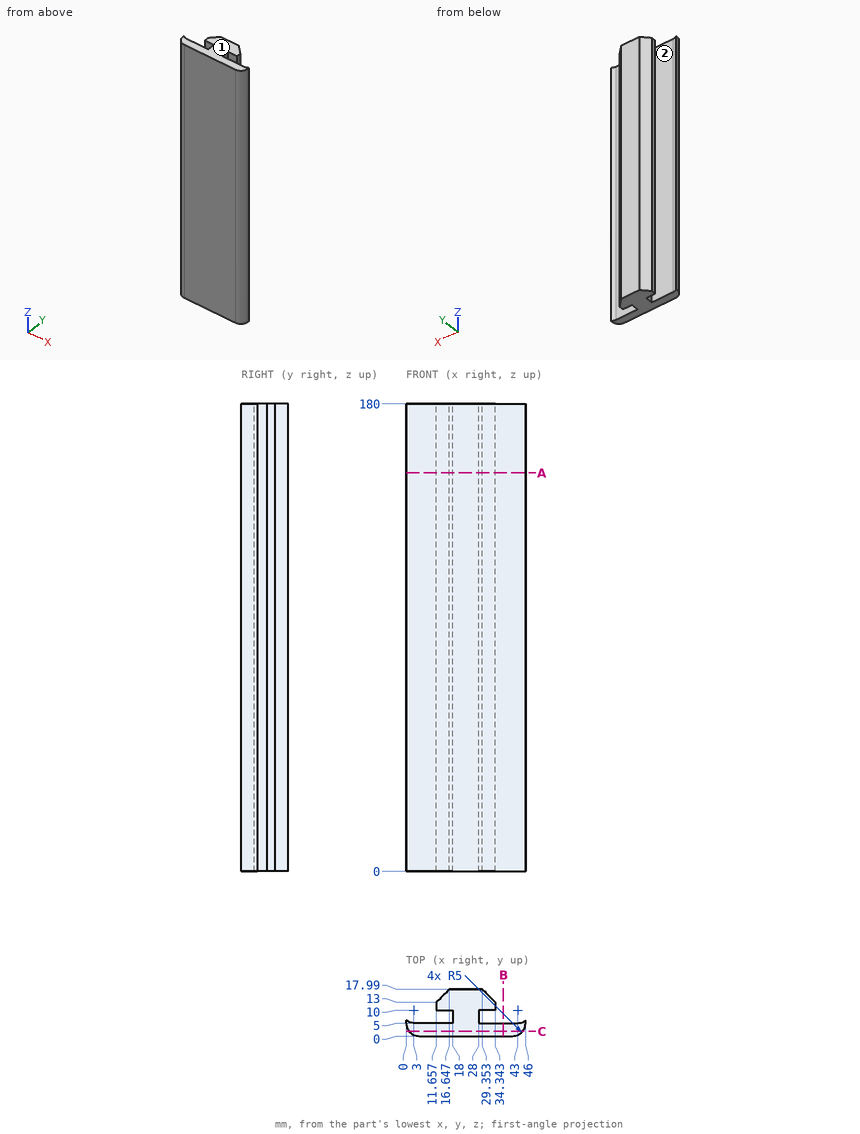
Source: three-view drawing plus pictorial views. Frame: mm from the lowest corner of the part. Round coordinates to 2 decimals unless told otherwise and drop trailing zeros. Loops run counter-clockwise (first coordinate to the right, second up) from the corner with the lowest first, then second, coordinate; pieces in that order, holes last.
Q1. Section B-B, the plane x = 37.5. Return loops of the section in (y, z), plus the area to 3 significant figures.
Q2. Section C-C, the plane y = 1.75. Return loops of the section in (x, z).
Q3. Mould query, pull axis X, two halves, no side actions, for the marked faces 1 and 2. Classes: pulls with the +X half, pulls with the -X half, needs draft (parallel to the pull), parting line crosses it, or undercut.
Q4. First-contact query: P1, Ø12, axis at x = 12, z = 111, coming from the +Y side; P2, Ø4.5, axis at x = 35.5, z = 116, coming from the +Y side; P3, Ø1.5, axis at y = 11.5, z = 116.5, coming from the +X side; P4, Ø2, axis at y = 2.5, z = 23.5, coming from the -X side. Flat tips, straight axial feed; report the tip coordinate or a pass-through.
Q5. Section A-A, the plane z = 153.5. Return loops of the section in (x, y).
Q6. Ray query, line 1 (Y direction, x = 28.5, z = 46); line 2 (X direction, y = 12.5, z = 128); line 3 (Y direction, x = 38.5, z = 127.5). Return the intervals inside material, ascending.
Solutions:
1. outline: (0, 0) - (5, 0) - (5, 180) - (0, 180) - close
1. area: 900 mm2
2. outline: (1.2, 0) - (44.8, 0) - (44.8, 180) - (1.2, 180) - close
3. face 1: needs draft
3. face 2: undercut
4. P1: stops at y = 17.99
4. P2: stops at y = 14.09
4. P3: stops at x = 34.34
4. P4: stops at x = 0.23
5. outline: (0, 5) arc R5 ccw to (5, 0) - (41, 0) arc R5 ccw to (46, 5) - (46, 6) arc R5 cw to (43, 5) - (28, 5) - (28, 10) - (34.34, 10) - (34.34, 13) - (29.35, 17.99) - (16.65, 17.99) - (11.66, 13) - (11.66, 10) - (18, 10) - (18, 5) - (3, 5) arc R5 cw to (0, 6) - close
6. line 1: y = 0 to 5, 10 to 17.99
6. line 2: x = 11.66 to 34.34
6. line 3: y = 0 to 5
